from build123d import *

# Parameters (mm, degrees)
F0_W           = 30
F0_H           = 145
F1_DEPTH       = 8
F2_D           = 3
F3_D           = 0.1
F3_DEPTH       = 23
F3_CBORE_D     = 10
F3_CBORE_DEPTH = 3
F3_TIP         = 0.030043031
F4_SIZE        = 5


with BuildPart() as f1:
    # F0 (on Front) → F1 (new body)
    with BuildSketch(Plane.XZ):
        with Locations((-5.6524093151, 12.860655725)):
            Rectangle(F0_W, F0_H)
    extrude(amount=F1_DEPTH)

    # F2 (through all)
    with Locations(Plane(origin=(0, 0, 0), x_dir=(1, 0, 0), z_dir=(0, 1, 0))):
        with Locations((5.3475906849, -76.360655725), (5.3475906849, -50.960655725), (5.3475906849, -25.560655725), (5.3475906849, -0.160655725), (5.3475906849, 25.239344275), (5.3475906849, 50.639344275), (-16.6524093151, 50.639344275), (-16.6524093151, 25.239344275), (-16.6524093151, -0.160655725), (-16.6524093151, -25.560655725), (-16.6524093151, -50.960655725), (-16.6524093151, -76.360655725)):
            Hole(F2_D / 2)

    # F3
    with Locations(Plane(origin=(0, 0, 0), x_dir=(1, 0, 0), z_dir=(0, 1, 0))):
        with Locations((-5.6524093151, -76.360655725), (-5.6524093151, -50.960655725), (-5.6524093151, -25.560655725), (-5.6524093151, -0.160655725), (-5.6524093151, 25.239344275), (-5.6524093151, 50.639344275)):
            CounterBoreHole(F3_D / 2, F3_CBORE_D / 2, F3_CBORE_DEPTH, depth=F3_DEPTH)
            with Locations((0, 0, -(F3_DEPTH + F3_TIP / 2))):  # 118° drill point
                Cone(0, F3_D / 2, F3_TIP, mode=Mode.SUBTRACT)

    # F4
    f4_edges = [f1.edges().sort_by_distance(p)[0] for p in [
        (9.347591, -4, -59.639344),
        (-20.652409, -4, -59.639344),
        (-20.652409, -4, 85.360656),
        (9.347591, -4, 85.360656),
    ]]
    chamfer(f4_edges, length=F4_SIZE)


solid = f1.part
Work out the finished part from the listing and answer in its coordinate system (mm). A direction names the side the tool comes from. Coordinates: 2 decimals unless noted, no trailing zeros. Write each loop counter-clockwise with the first axis right and the second up, starting at its lowest first coordinate (ties: lowest second). Pieces come first, ordered by that corner, then holes. Notation, with made-up numbers: M -37,-3.75 L 5,-3.75 A18 cw 5,0.25 Z; hole C -13.5,-28 d5. An arc over 180 degrees is marked long. Write item = value, one per line.
1. The part is cut by section C-C (z = -47.5). Determine the outline of the cut face in (x, y).
Solution:
outline = M -20.65,-8 L 9.35,-8 L 9.35,0 L -1.76,0 L -1.76,-3 L -9.54,-3 L -9.54,0 L -20.65,0 Z
2. For faces 1 (the face through (-18.12, -3.94, -57.17)), 2 (the face through (-6.303, -1.479, -55.597)), determine the directions among +Z, -Z, +X, -X, +Y, -Y from which every point of the face is accessible in a straight line to the end or side of a thin tool.
Solution:
face_1 = -Z, -X, +Y, -Y
face_2 = +Y
3. Determine the mould class of faces 3 (the face through (-6, 0, 14)), 4 (the face through (6.88, -3.94, 82.83)), 5 (the face through (-15.154, -4.056, 0.095)), 6 (the face through (-6, -4, -59.639)) for opening direction Z: released by +Z, released by -Z, zero draft, split by the parting line, or undercut.
Solution:
face_3 = zero draft
face_4 = released by +Z
face_5 = undercut
face_6 = released by -Z
4. The part is cut by section A-A (y = -5.5). State how many separate pieces and enclosed holes the cut face has, then the cut area to 3 significant figures.
Solution:
separate_pieces = 1
enclosed_holes = 18
area = 4,220 mm2
5. The part is cut by section B-B (x = -2). Determine the outline of the cut face in (y, z), then the cut area to 3 significant figures.
Solution:
outline = M -8,-59.64 L 0,-59.64 L 0,-54.05 L -3,-54.05 L -3,-47.22 L 0,-47.22 L 0,-28.65 L -3,-28.65 L -3,-21.82 L 0,-21.82 L 0,-3.25 L -3,-3.25 L -3,3.58 L 0,3.58 L 0,22.15 L -3,22.15 L -3,28.98 L 0,28.98 L 0,47.55 L -3,47.55 L -3,54.38 L 0,54.38 L 0,72.95 L -3,72.95 L -3,79.78 L 0,79.78 L 0,85.36 L -8,85.36 Z
area = 1,040 mm2
6. Flat-ended cylindrical pins translate along their axes: pin 1 (2.5 mm diameter, centred on x = -16.65, z = -25.24, fed in from +Y); pin 2 (8 mm diameter, centred on x = -5.65, z = -50.64, fed in from +Y). Find the tip coordinate at first contact, or state that the pin passes through.
Solution:
pin_1 = through
pin_2 = -3
7. Straight lines are drawn through the part: line 1 (X direction, y = -2, z = -52); line 2 (X direction, y = -0.25, z = -0.5); line 3 (Y direction, x = -4.25, z = 25.5). For each, find the intervals that lie inside material, in ascending order. Write a range as from..to.
Solution:
line_1 = -20.65..-17.28, -16.02..-10.46, -0.84..4.72, 5.98..9.35
line_2 = -20.65..-18, -15.31..-10.61, -0.7..4, 6.69..9.35
line_3 = -8..-3
